The model under review builds one solid part; all positions refer to its coordinate system, in mm. Face numbers are marked on the shaded views. A direction names the side the tool comes from. Coordinates: 2 decimals unless noted, no trailing zeros. Order: outer loops, then holes, each group sorted by start corner. A loop starts at its lowest first (then second) coordinate and runs counter-clockwise, first axis right, second up. Notation, with made-up numbers: M -3.5,-4 L 41.5,-4 A16 ccw 41.5,12 Z; hole C 14,46.25 d2. An arc over 180 degrees is marked long. One line per item, written item: value.
Autodesk Inventor part; units mm, degrees
ref_plane "YZ Plane" through (0, 0, 0) normal (1, 0, 0) x (0, 1, 0)
ref_plane "XZ Plane" through (0, 0, 0) normal (0, 1, 0) x (-1, 0, 0)
ref_plane "XY Plane" through (0, 0, 0) normal (0, 0, 1) x (1, 0, 0)
sketch "Sketch1" plane through (0, 0, 0) normal (0, 0, 1) x (1, 0, 0)
  line L0 (-36.9504, 0) -> (-18.4752, 32)
  line L1 (-18.4752, 32) -> (18.4752, 32)
  line L2 (18.4752, 32) -> (36.9504, 0)
  line L3 (36.9504, 0) -> (18.4752, -32)
  line L4 (18.4752, -32) -> (-18.4752, -32)
  line L5 (-18.4752, -32) -> (-36.9504, 0)
  circle A0 centre (0, 0) radius 12
  dimension "d0" = 64
  dimension "d1" = 24
extrude "Extrusion1" add sketch "Sketch1" along normal blind 13
sketch "Sketch2" plane through (0, 0, 0) normal (0, 0, -1) x (-1, 0, 0)
  line L0 (68.1273, 0) -> (34.0637, -59)
  line L1 (34.0637, -59) -> (-34.0637, -59)
  line L2 (-34.0637, -59) -> (-68.1273, 0)
  line L3 (-68.1273, 0) -> (-34.0637, 59)
  line L4 (-34.0637, 59) -> (34.0637, 59)
  line L5 (34.0637, 59) -> (68.1273, 0)
  circle A0 centre (0, 0) radius 12
  line L6 (68.1273, 0) -> (68.1273, 149)
  line L7 (68.1273, 149) -> (-68.1273, 149)
  line L8 (-68.1273, 149) -> (-68.1273, 0)
  dimension "d4" = 118
  dimension "d8" = 90
extrude "Extrusion2" add sketch "Sketch2" along normal blind 200
sketch "Sketch3" plane through (0, 0, -200) normal (0, 0, -1) x (-1, 0, 0)
  circle A0 centre (0, 0) radius 12
extrude "Extrusion3" add sketch "Sketch3" against normal blind 120
sketch "Sketch4" plane through (0, 0, 0) normal (0, 0, 1) x (1, 0, 0)
  line L0 (68.1273, 0) -> (34.0637, -59)
  line L1 (34.0637, -59) -> (-34.0637, -59) construction
  line L2 (-34.0637, -59) -> (-68.1273, 0)
  line L3 (-68.1273, 0) -> (-34.0637, 59)
  line L4 (-34.0637, 59) -> (34.0637, 59)
  line L5 (34.0637, 59) -> (68.1273, 0)
  line L6 (68.1273, 0) -> (34.0637, -59)
  line L7 (68.1273, 149) -> (68.1273, 0)
  line L8 (68.1273, 0) -> (68.1273, 149)
  line L9 (-68.1273, 149) -> (68.1273, 149)
  line L10 (68.1273, 149) -> (-68.1273, 149)
  line L11 (-68.1273, 149) -> (-68.1273, 0)
  point P0 (0, 0)
  point P1 (0, 0)
extrude "Extrusion4" cut sketch "Sketch4" against normal blind 50
chamfer "Chamfer1" distance 125 angle 45 1 edges at (0, -59, -200)
chamfer "Chamfer2" distance 34 angle 45 2 edges at (-68.1273, 33, -167) (68.1273, 33, -167)
sketch "Sketch5" plane through (-68.1273, 149, -200) normal (0, 1, 0) x (1, 0, 0)
  line L0 (0, -150) -> (0, 0)
  line L1 (0, 0) -> (-30, 0)
  line L2 (-30, 0) -> (-30, -150)
  line L3 (-30, -150) -> (0, -150)
  line L4 (0, -150) -> (0, 0)
  line L5 (0, 0) -> (136.2547, 0)
  line L6 (136.2547, 0) -> (166.2547, 0)
  line L7 (166.2547, 0) -> (166.2547, -150)
  line L8 (166.2547, -150) -> (136.2547, -150)
  line L9 (136.2547, -150) -> (136.2547, 0)
  circle A0 centre (151.2547, -131) radius 3
  circle A1 centre (151.2547, -103) radius 3
  circle A2 centre (151.2547, -75) radius 3
  circle A3 centre (151.2547, -47) radius 3
  circle A4 centre (151.2547, -19) radius 3
  line L10 (68.1273, -200) -> (68.1273, -239.5833)
  line L11 (0, 0) -> (-30, 0)
  line L12 (-30, 0) -> (-30, -150)
  line L13 (-30, -150) -> (0, -150)
  line L14 (0, -150) -> (0, 0)
  circle A5 centre (-15, -131) radius 3
  circle A6 centre (-15, -103) radius 3
  circle A7 centre (-15, -75) radius 3
  circle A8 centre (-15, -47) radius 3
  circle A9 centre (-15, -19) radius 3
  point P0 (151.2547, -150)
  point P1 (0, -150)
  point P2 (-15, -150)
  dimension "d19" = 30
  dimension "d20" = 30
  dimension "d21" = 6
  dimension "d22" = 19
  dimension "d25" = 28
extrude "Extrusion5" add sketch "Sketch5" against normal blind 25
chamfer "Chamfer4" distance 10 angle 45 4 edges at (98.1273, 136.5, -50) (-98.1273, 136.5, -50) (98.1273, 136.5, -200) (-98.1273, 136.5, -200)
properties part number "BA30" material "ABS Plastic"
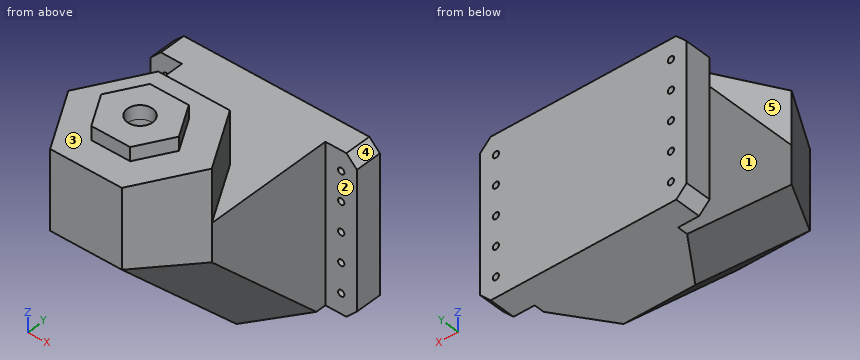
(1) Tool access review of the marked faces 1, 2, 3, 4 and 5: name each direction out of +Z, -Z, +X, -X, +Y, -Y from which nothing blocks a thin tool from reaching the whole face with its end or side.
Geometry results:
face 1: +Z, -Z, -X, -Y
face 2: +Z, -Z, +X, -Y
face 3: +Z
face 4: +Z, +X, +Y, -Y
face 5: +Z, -X, +Y
(2) We need section C-C, the plane x = 0. State the section outline as (y, z) points, plus the area to 3 significant figures.
Geometry results:
outline: M -59,-75 L 66,-200 L 149,-200 L 149,-50 L 59,-50 L 59,0 L 32,0 L 32,13 L 12,13 L 12,-80 L -12,-80 L -12,13 L -32,13 L -32,0 L -59,0 Z
area: 27,900 mm2
(3) For L1, parallel to X at y = 136.75, z = -69; L2, parallel to Y at x = 70, z = -55; L3, parallel to X at y = 90, z = -136.5, list the stretches that pass through material, from the lowest coordinate up.
Geometry results:
L1: x = -98.13 to -86.13, -80.13 to 80.13, 86.13 to 98.13
L2: y = 124 to 149
L3: x = -68.13 to 68.13
(4) We need section A-A, the plane z = -69. State the section outline as (x, y) points, plus the area to 3 significant figures.
Geometry results:
outline: M -98.13,124 L -86.13,124 L -86.13,149 L -98.13,149 Z; M -80.13,124 L -68.13,124 L -68.13,0 L -34.06,-59 L 34.06,-59 L 68.13,0 L 68.13,124 L 80.13,124 L 80.13,149 L -80.13,149 Z; M 86.13,124 L 98.13,124 L 98.13,149 L 86.13,149 Z; hole C 0,0 d24
area: 27,100 mm2
(5) We need section B-B, the plane z = -125. State the section outline as (x, y) points, plus the area to 3 significant figures.
Geometry results:
outline: M -98.13,124 L -86.13,124 L -86.13,149 L -98.13,149 Z; M -80.13,124 L -68.13,124 L -68.13,39.08 L -34.13,-9 L 34.13,-9 L 68.13,39.08 L 68.13,124 L 80.13,124 L 80.13,149 L -80.13,149 Z; M 86.13,124 L 98.13,124 L 98.13,149 L 86.13,149 Z
area: 21,100 mm2
(6) Insertion check: pin 1 Ø9 at (x, z) = (-77, -98.5) entering from -Y; pin 2 Ø1.5 at (y, z) = (33, -98.5) entering from +X; pin 3 Ø4 at (x, y) = (33.5, 63) entering from -Z. Each pin has a flat end and moves straight along its axis. Give the tip position at first contact, or say it passes through.
Geometry results:
pin 1: stops at y = 124
pin 2: stops at x = 68.13
pin 3: stops at z = -199
(7) We need section D-D, the plane y = -5. State the section outline as (x, z) points, plus the area to 3 significant figures.
Geometry results:
outline: M -65.24,-85 L -34.13,-129 L 34.13,-129 L 65.24,-85 L 65.24,0 L 34.06,0 L 34.06,13 L 10.91,13 L 10.91,-80 L -10.91,-80 L -10.91,13 L -34.06,13 L -34.06,0 L -65.24,0 Z
area: 14,300 mm2
